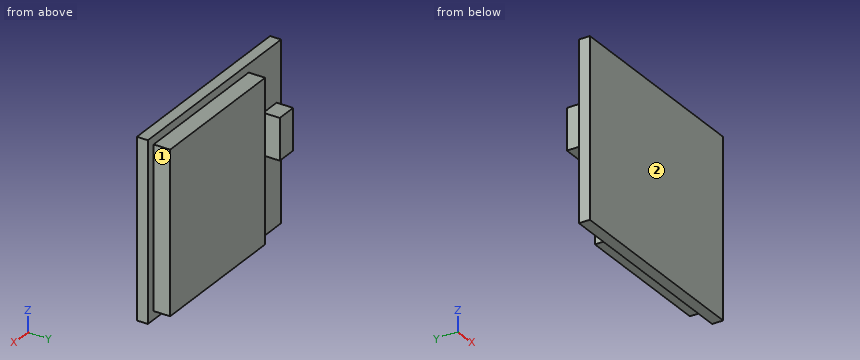
from build123d import *

# Parameters (mm, degrees)
SKETCH1_W           = 15
SKETCH1_H           = 12.9
BOSS_EXTRUDE1_DEPTH = 0.4
SKETCH2_W           = 10.7
SKETCH2_H           = 11.7
BOSS_EXTRUDE2_DEPTH = 1.2
SKETCH3_W           = 1.5
SKETCH3_H           = 3
BOSS_EXTRUDE3_DEPTH = 1.2


with BuildPart() as part:
    # Sketch1 → Boss-Extrude1 (new body, symmetric)
    with BuildSketch(Plane(origin=(0, 0, 0), x_dir=(1, 0, 0), z_dir=(0, 1, 0))):
        Rectangle(SKETCH1_W, SKETCH1_H)
    extrude(amount=BOSS_EXTRUDE1_DEPTH, both=True)

    # Sketch2 → Boss-Extrude2 (add)
    with BuildSketch(Plane(origin=(0, 0.4, 0), x_dir=(1, 0, 0), z_dir=(0, 1, 0))):
        with Locations((1.5, 0)):
            Rectangle(SKETCH2_W, SKETCH2_H)
    extrude(amount=BOSS_EXTRUDE2_DEPTH)

    # Sketch3 → Boss-Extrude3 (add)
    with BuildSketch(Plane(origin=(0, 0.4, 0), x_dir=(1, 0, 0), z_dir=(0, 1, 0))):
        with Locations((-6.25, -0.75)):
            Rectangle(SKETCH3_W, SKETCH3_H)
    extrude(amount=BOSS_EXTRUDE3_DEPTH)


solid = part.part
Build history of the part. All positions in model axes, mm. Face numbers are marked on the shaded views. A direction names the side the tool comes from. Give positions to 0.01 mm unless a question says otherwise; leave off trailing zeros. Order: outer loops, then holes, each group sorted by start corner. A loop starts at its lowest first (then second) coordinate and runs counter-clockwise, first axis right, second up. Notation, with made-up numbers: M 43,-0.5 L 85,-0.5 A18 ccw 85,13.5 Z; hole C 87.25,45 d7. An arc over 180 degrees is marked long. Use one line per item in the form item = value.
Q1. Pin check, flat tips, straight feed: P1, Ø0.6, axis at x = 0.5, y = 1, coming from the +Z side; P2, Ø0.6, axis at y = 1, z = 2, coming from the -X side; P3, Ø1, axis at y = 1, z = 1.5, coming from the +X side. Stop position of each tip, or through.
Conclusion:
P1 = 5.85
P2 = -7
P3 = 6.85
Q2. Slice it at B-B, the plane z = 3.5. Write the cut outline in (x, y).
Conclusion:
outline = M -7.5,-0.4 L 7.5,-0.4 L 7.5,0.4 L 6.85,0.4 L 6.85,1.6 L -3.85,1.6 L -3.85,0.4 L -7.5,0.4 Z
Q3. Slice it at C-C, the plane x = 0.5. Write the cut outline in (y, z), and give its area (3 significant figures).
Conclusion:
outline = M -0.4,-6.45 L 0.4,-6.45 L 0.4,-5.85 L 1.6,-5.85 L 1.6,5.85 L 0.4,5.85 L 0.4,6.45 L -0.4,6.45 Z
area = 24.4 mm2
Q4. Slice it at D-D, the plane z = 1. Write the cut outline in (x, y).
Conclusion:
outline = M -7.5,-0.4 L 7.5,-0.4 L 7.5,0.4 L 6.85,0.4 L 6.85,1.6 L -3.85,1.6 L -3.85,0.4 L -5.5,0.4 L -5.5,1.6 L -7,1.6 L -7,0.4 L -7.5,0.4 Z
Q5. Wall check: probe 1 along X at (y, z) = (1.15, 1); probe 2 along Z at (x, y) = (-6.75, 0.8); probe 3 along X at (y, z) = (0.95, -2.5). Give the ranges that are in metal, low to high.
Conclusion:
probe_1 = -7 to -5.5, -3.85 to 6.85
probe_2 = -0.75 to 2.25
probe_3 = -3.85 to 6.85
Q6. Which spindle directions (+Z, -Z, +X, -X, +Y, -Y) get a long thin tool onto all of the face, cutting with end or side? Do the marked faces 1 and 2. Say none if no direction does.
Conclusion:
face_1 = +Z, -Z, +X, +Y
face_2 = +Z, -Z, +X, -X, -Y
Q7. Slice it at A-A, the plane y = 0.85. Write the cut outline in (x, z), and give its area (3 significant figures).
Conclusion:
outline = M -7,-0.75 L -5.5,-0.75 L -5.5,2.25 L -7,2.25 Z; M -3.85,-5.85 L 6.85,-5.85 L 6.85,5.85 L -3.85,5.85 Z
area = 130 mm2
